Here's how the part is built. I have some questions about the finished solid (model axes, mm). A direction names the side the tool comes from. Round coordinates to 2 decimals unless told otherwise and drop trailing zeros. Order: outer loops, then holes, each group sorted by start corner. A loop starts at its lowest first (then second) coordinate and runs counter-clockwise, first axis right, second up. Notation, with made-up numbers: (34.25, 5.25) - (73.25, 5.25) arc R20 cw to (73.25, 17.25) - close; hole circle Ø4 at (5, 22.25). An arc over 180 degrees is marked (long way). One line per item, written item: value.
from build123d import *
from build123d.topology import SkipClean

# Parameters (mm, degrees)
SKETCH1_R                = 32.5
BOSS_EXTRUDE1_DEPTH      = 5
BOSS_EXTRUDE2_DEPTH      = 15
BOSS_EXTRUDE2_DEPTH_BACK = 5
BOSS_EXTRUDE2_START      = 5
SKETCH2_R                = 30.5
CUT_EXTRUDE3_START       = 10
SKETCH3_R                = 24
CUT_EXTRUDE3_DEPTH       = 41.124844139
CUT_EXTRUDE3_DRAFT       = -12
FILLET1_R                = 4
SKETCH4_R                = 24
CUT_EXTRUDE4_DEPTH       = 49.347699015
FILLET2_R                = 12
SKETCH5_R                = 28
SKETCH5_R_2              = 24
BOSS_EXTRUDE3_DEPTH      = 23
FILLET3_R                = 0.5


with BuildPart() as part:
    # Sketch1 → Boss-Extrude1 (new body)
    with BuildSketch(Plane(origin=(0, 0, 0), x_dir=(1, 0, 0), z_dir=(0, 1, 0))):
        with Locations(Location((0, 0, 0), (0, 0, 270))):
            Circle(SKETCH1_R)
    extrude(amount=BOSS_EXTRUDE1_DEPTH)

    # Sketch2 → Boss-Extrude2 (add, two sides: drawn at the far end of the back side and taken through both)
    with BuildSketch(Plane.XZ.offset(BOSS_EXTRUDE2_START - BOSS_EXTRUDE2_DEPTH_BACK)):
        with Locations(Location((0, 0, 0), (0, 0, 270))):
            Circle(SKETCH2_R)
    extrude(amount=BOSS_EXTRUDE2_DEPTH + BOSS_EXTRUDE2_DEPTH_BACK)


with BuildPart() as cut_extrude3_tool:
    # Sketch3 → Cut-Extrude3 (with draft: the straight prism first)
    with BuildSketch(Plane(origin=(0, 0, 0), x_dir=(-1, 0, 0), z_dir=(0, -1, 0)).offset(CUT_EXTRUDE3_START)):
        Circle(SKETCH3_R)
    extrude(amount=CUT_EXTRUDE3_DEPTH)
    # Cut-Extrude3: the draft: its side faces are tilted about the plane it starts from
    cut_extrude3_sides = [cut_extrude3_tool.faces().sort_by_distance(p)[0] for p in [
        (24, -30.56242207, 0),
    ]]
    draft(cut_extrude3_sides, Plane(origin=(0, 0, 0), x_dir=(-1, 0, 0), z_dir=(0, -1, 0)).offset(CUT_EXTRUDE3_START), CUT_EXTRUDE3_DRAFT)


with BuildPart() as part_1:
    add(part.part)

    # Cut-Extrude3: cut by cut_extrude3_tool
    add(cut_extrude3_tool.part, mode=Mode.SUBTRACT)

    # Fillet1
    fillet1_edges = [part_1.edges().sort_by_distance(p)[0] for p in [
        (26.125565617, -20, 0),
    ]]
    fillet(fillet1_edges, radius=FILLET1_R)

    # Sketch4 → Cut-Extrude4 (cut, through all)
    with BuildSketch(Plane.XZ.offset(10)):
        with Locations(Location((0, 0, 0), (0, 0, 270))):
            Circle(SKETCH4_R)
    extrude(amount=-CUT_EXTRUDE4_DEPTH, mode=Mode.SUBTRACT)

    # Fillet2
    fillet2_edges = [part_1.edges().sort_by_distance(p)[0] for p in [
        (-16.970562748, -10, -16.970562748),
    ]]
    fillet(fillet2_edges, radius=FILLET2_R)

    # Sketch5 → Boss-Extrude3 (add)
    with SkipClean():  # the faces are left unmerged after this step: merging them gives an invalid solid
        with BuildSketch(Plane(origin=(0, 5, 0), x_dir=(1, 0, 0), z_dir=(0, 1, 0))):
            with Locations(Location((0, 0, 0), (0, 0, 270))):
                Circle(SKETCH5_R)
            with Locations(Location((0, 0, 0), (0, 0, 270))):
                Circle(SKETCH5_R_2, mode=Mode.SUBTRACT)
        extrude(amount=BOSS_EXTRUDE3_DEPTH)
    add(part_1.part.scale(1), mode=Mode.REPLACE)  # the faces are merged on a copy

    # Fillet3
    fillet3_edges = [part_1.edges().sort_by_distance(p)[0] for p in [
        (0, 28, -28),
        (0, 28, -24),
    ]]
    fillet(fillet3_edges, radius=FILLET3_R)


solid = part_1.part
Q1. If I drill on line 1 along X through (y, z) = (-4, 0); line 2 along X through (y, z) = (13.5, 0); line 3 along Z through (x, y) = (-10, 19), over which ranges is the centre line in solid material (lowest first)?
Results list:
line 1: -30.5 to -24, 24 to 30.5
line 2: -28 to -24, 24 to 28
line 3: -26.15 to -21.82, 21.82 to 26.15
Q2. We'd pull the mould along X, two halves only. Please class faces 4 (the flat face through (25, -20, 16)), 5 (the conical face through (-11.22, -11.51, 21.58)), 6 (the cylindrical face through (-29.775, -9.86, 6.612)): released by +X, released by -X, zero draft, split by the parting line, or undercut.
Results list:
face 4: zero draft
face 5: undercut
face 6: split by the parting line
Q3. If we section it at B-B, the plane y = -2: Please give me the cut outline in (x, z).
Results list:
outline: circle Ø61 at (0, 0); hole circle Ø48 at (0, 0)
Q4. Which directions (+Z, -Z, +X, -X, +Y, -Y) give clear straight access to the entire face, cutting with the end or side of a thin tool? Please do faces 1 (the flat face through (29, 0, -10)), 2 (the flat face through (-2, 28, -25)), 3 (the cylindrical face through (-27.334, 16.093, -6.07)).
Results list:
face 1: -Y
face 2: +Z, -Z, +X, -X, +Y
face 3: +Y
Q5. If we section it at A-A, the plane y = 17: Please give me the cut outline in (x, z), then the cut area to 3 significant figures.
Results list:
outline: circle Ø56 at (0, 0); hole circle Ø48 at (0, 0)
area: 653 mm²
Q6. Will these pins go through, and if not, where does the flat tip stop? pin 1 (4 mm diameter, centred on y = -4.5, z = 2, fed in from +X); pin 2 (6 mm diameter, centred on x = 24.5, z = 10.5, fed in from -Y); pin 3 (4 mm diameter, centred on x = 8, y = 10.5, fed in from +Z); pin 4 (1 mm diameter, centred on x = 19.5, y = 21.5, fed in from +Z).
Results list:
pin 1: x = 30.5
pin 2: y = -20
pin 3: z = 27.35
pin 4: z = 20.57
